Input: part model. Units: mm. Frame: model coordinates. Round coordinates to 2 decimals unless told otherwise and drop trailing zeros. Loops run counter-clockwise (first coordinate to the right, second up) from the corner with the lowest first, then second, coordinate; pieces in that order, holes last. Notation, with made-up numbers: (-13, 28.5) -> (44, 28.5) arc R18 ccw to (44, 39.5) -> close; hole circle Ø7 at (45, 30). An arc over 180 degrees is marked (long way). One line per question, with ' | ' between items. Start each with the question number.
Q1. Cut plane B-B on y = 360.5. Return loops of the section in (x, z).
Q2. Material intervals for L1, parallel to Y at x = 3.5, z = 1611.5; L2, parallel to Y at x = 3.05, z = 1613; L3, parallel to Y at x = 3.1, z = 1622, sorted ascending.
Q3. Cut plane A-A on x = 2.55. Return loops of the section in (y, z).
Q4. Cut plane C-C on z = 1602. Return loops of the section in (x, y), and give its area (3 significant figures).
Q5. Contact query for flat-ended pins moving along their axis: P1, Ø8, axis at y = 352.04, z = 1608.48, coming from the -X side; P2, Ø2, axis at x = 4, z = 1632.5, coming from the +Y side. Output: stop coordinate, or through.
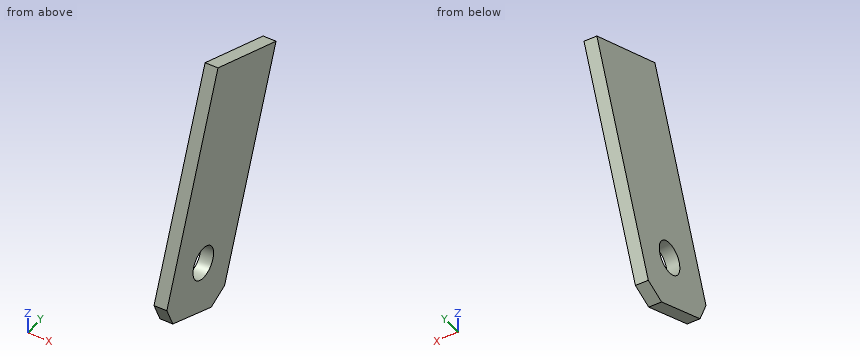
from build123d import *

# Parameters (mm, degrees)
BOSS_EXTRUDE1_DEPTH  = 4
M8_CLEARANCE_HOLE1_D = 9.999053744
CHAMFER1_SIZE        = 5


with BuildPart() as part:
    # Sketch1 → Boss-Extrude1 (new body)
    with BuildSketch(Plane(origin=(0.900000083, 0, 0), x_dir=(0, -1, 0), z_dir=(-1, 0, 0))):
        Polygon((-360.573996926, 1589.166586834), (-332.547614774, 1599.868077547), (-359.157201755, 1669.556541862), (-387.327723707, 1659.232542214), align=None)
    extrude(amount=-BOSS_EXTRUDE1_DEPTH)

    # M8 Clearance Hole1 (through all)
    with Locations(Plane(origin=(4.900000083, 0, 0), x_dir=(0, 0, -1), z_dir=(1, 0, 0))):
        with Locations((-1608.483107892, 352.03572843)):
            Hole(M8_CLEARANCE_HOLE1_D / 2)

    # Chamfer1
    chamfer1_edges = [part.edges().sort_by_distance(p)[0] for p in [
        (2.900000083, 332.547614774, 1599.868077547),
        (2.900000083, 360.573996926, 1589.166586834),
    ]]
    chamfer(chamfer1_edges, length=CHAMFER1_SIZE)


solid = part.part
Results:
1) outline: (0.9, 1593.01) -> (4.9, 1593.01) -> (4.9, 1669.06) -> (0.9, 1669.06) -> close
2) L1: 336.99 to 348.05, 356.02 to 369.1 | L2: 337.56 to 349.89, 354.18 to 369.67 | L3: 341 to 373.11
3) outline: (334.33, 1604.54) -> (337.22, 1598.08) -> (355.9, 1590.95) -> (362.36, 1593.84) -> (387.33, 1659.23) -> (359.16, 1669.56) -> close; hole circle Ø10 at (352.04, 1608.48)
4) outline: (0.9, 335.47) -> (4.9, 335.47) -> (4.9, 365.47) -> (0.9, 365.47) -> close | area: 120 mm^2
5) P1: through | P2: y = 377.5
